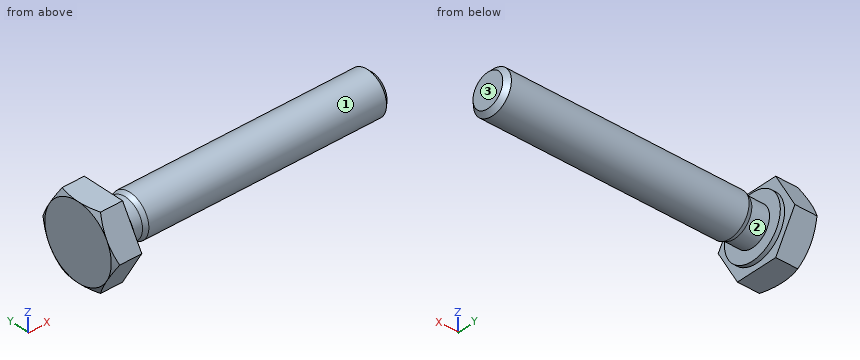
Autodesk Inventor part; units mm, degrees
ref_plane "Work Plane1" through (1.525, 0, 0) normal (0, 0, 1) x (1, 0, 0)
ref_plane "YZ Plane" through (0, 0, 0) normal (1, 0, 0) x (0, 1, 0)
ref_plane "XZ Plane" through (0, 0, 0) normal (0, 1, 0) x (-1, 0, 0)
sketch "Skizze1" plane through (0, 0, 0) normal (0, 0, 1) x (1, 0, 0)
  line L0 (0, 2.95) -> (0, 1.8106)
  line L1 (2.1, 2) -> (25, 2)
  line L2 (25, 2) -> (25, 0)
  line L3 (25, 0) -> (-0.4001, 0)
  line L4 (-5.4801, 0) -> (30.08, 0)
  line L5 (-0.4001, 0) -> (-0.4001, 2.95)
  line L6 (-0.4001, 2.95) -> (0, 2.95)
  line L7 (2.1, 2) -> (1.6705, 1.8106)
  line L8 (1.6705, 1.8106) -> (0, 1.8106)
  line L9 (0, -0.59) -> (0, 3.54)
  dimension "d0" = 25
  dimension "d1" = 22.9
  dimension "d2" = 4
  dimension "d9" = 0.4001
  dimension "d10" = 5.9
  dimension "d13" = 0.4295
  dimension "d14" = 3.6211
revolve "Körper" add sketch "Skizze1" angle 360 about axis through (25, 0, 0) along (-1, 0, 0)
sketch "Skizze2" plane through (-0.4001, 0, 0) normal (-1, 0, 0) x (0, 0, 1)
  line L0 (0, 4.0415) -> (3.5, 2.0207)
  line L1 (3.5, 2.0207) -> (3.5, -2.0207)
  line L2 (3.5, -2.0207) -> (0, -4.0415)
  line L3 (0, -4.0415) -> (-3.5, -2.0207)
  line L4 (-3.5, -2.0207) -> (-3.5, 2.0207)
  line L5 (-3.5, 2.0207) -> (0, 4.0415)
  point P0 (0, 0)
  point P1 (0, 0)
  dimension "d11" = 7
extrude "Kopf" add sketch "Skizze2" along normal blind 2.4
sketch "Skizze4" plane through (0, 0, 0) normal (0, 0, 1) x (1, 0, 0)
  line L0 (-2.8001, 3.5) -> (-2.8001, 4.0415)
  line L1 (-2.8001, 4.0415) -> (-2.4875, 4.0415)
  line L2 (-2.4875, 4.0415) -> (-2.8001, 3.5)
  line L3 (-3.2801, 0) -> (0.0799, 0)
  line L4 (-0.4001, 4.0415) -> (-2.8001, 4.0415)
  line L5 (-2.8001, 2.0207) -> (-2.8001, 4.0415)
  dimension "d5" = 30
  dimension "d19" = 7
revolve "Fase1" cut sketch "Skizze4" angle 360 about axis through (-10, 0, 0) along (1, 0, 0)
thread "Gewinde"
chamfer "Fase2" distance 0.4294 distance2 0.4295 1 edges at (25, -2, 0) measured on face at (25, -0.0804, -0.6618)
ref_plane "Work Plane1" through (1.525, 0, 0) normal (0, 0, 1) x (1, 0, 0)
equation "\"d0\" = NLG"
equation "\"d1\" = GEL"
equation "\"d2\" = GD"
equation "\"d10\" = SD2"
equation "\"d14\" = BDM"
equation "\"d11\" = SW"
equation "\"d3\" = KOH - SD"
equation "\"d5\" = ANG1"
equation "\"d19\" = SW0"
equation "\"d15\" = GEL"
equation "\"d6\" = -0.5 * SPD + 0.5 * GD"
equation "\"NLG\" = 25"
equation "\"GD\" = NND"
equation "\"BDM\" = 3.62111"
equation "\"KOH\" = 2.8"
equation "\"GEL\" = 22.9"
equation "\"SW\" = 7"
equation "\"SW0\" = 7"
equation "\"SPD\" = NND - 1.2269 * PTC"
equation "\"SD2\" = 5.9"
equation "\"SD\" = 0.4"
equation "\"ANG1\" = 30deg"
equation "\"GAL\" = 0.61345 * PTC"
equation "\"GUL\" = 0.61345 * PTC"
equation "\"RR\" = 0.2"
equation "\"GD1\" = THREADDIA - 1.2269 * PTC"
equation "\"THREADDIA\" = 4"
equation "\"TOA\" = 30deg"
equation "\"PTC\" = 0.7"
equation "\"NND\" = 4"
equation "\"E0\" = 1.155 * SW"
properties part number "DIN 933 - M4  x 25" material "Stahl, weich"
Source: CAD feature listing. Evaluate the final solid. Frame: model axes, mm. Face numbers are marked on the shaded views. A direction names the side the tool comes from. Round coordinates to 2 decimals unless told otherwise and drop trailing zeros. Loops run counter-clockwise (first coordinate to the right, second up) from the corner with the lowest first, then second, coordinate; pieces in that order, holes last.
1. Ray query, L1, parallel to X at y = 1, z = 2.25; L2, parallel to X at y = -1, z = -3; L3, parallel to Y at x = 4, z = 0. Return the intervals inside material, ascending.
2. Access query for the marked faces 1, 2 and 3. Directions: +Z, -Z, +X, -X, +Y, -Y. A direction counts if a zero-diameter tool reaches every point of the face in a straight line with its end or side. Return the directions, or none.
3. Contact query for flat-ended pins moving along their axis: pin 1 (2 mm diameter, centred on x = 18, y = -1.5, fed in from +Z); pin 2 (3 mm diameter, centred on x = 7.5, y = 1, fed in from -Z). Output: stop coordinate, or through.
4. Section query A-A on x = 3.5. Output: boundary loops of the cut face in (y, z).
Answers below:
1. L1: x = -2.8 to 0
1. L2: x = -2.8 to -0.4
1. L3: y = -2 to 2
2. face 1: +X
2. face 2: none
2. face 3: +Z, -Z, +X, +Y, -Y
3. pin 1: stops at z = 1.94
3. pin 2: stops at z = -2
4. outline: circle Ø4 at (0, 0)
